Build history of the part. All positions in model axes, mm. Round coordinates to 2 decimals unless told otherwise and drop trailing zeros. Write each loop counter-clockwise with the first axis right and the second up, starting at its lowest first coordinate (ties: lowest second). Pieces come first, ordered by that corner, then holes.
Item 1: Band-saw the part on C-C, the plane x = 142. Write the cut outline in (y, z), then the cut area to 3 significant figures.
Item 2: Drop flat-ended pins along their axis: pin 1 Ø5 at (y, z) = (-13, 14.5) entering from -X; pin 2 Ø3 at (y, z) = (13.5, 13.5) entering from +X. Give the stop position or say it passes through.
Item 3: Wall check: probe 1 along Y at (x, z) = (160, 17); probe 2 along X at (y, z) = (1, 15); probe 3 along X at (y, z) = (-2.5, 13). Give the ranges that are in metal, low to high.
Item 4: Band-saw the part on A-A, the plane x = -160. Write the cut outline in (y, z), then the cut area to 3 significant figures.
Item 5: Band-saw the part on D-D, the plane y = -12.5. Write the cut outline in (x, z), then the cut area to 3 significant figures.
Item 6: Band-saw the part on B-B, the plane z = 15.5. Write the cut outline in (x, y), then the cut area to 3 significant figures.
```python
from build123d import *

# Parameters (mm, degrees)
SKETCH1_W           = 350
SKETCH1_H           = 35
BOSS_EXTRUDE1_DEPTH = 20
SKETCH2_W           = 80
SKETCH2_H           = 20
CUT_EXTRUDE1_DEPTH  = 178.006355818
SKETCH4_R           = 7.5
CUT_EXTRUDE2_DEPTH  = 178.006355818
FILLET1_R           = 10
FILLET2_R           = 10


with BuildPart() as part:
    # Sketch1 → Boss-Extrude1 (new, symmetric)
    with BuildSketch(Plane.XY):
        Rectangle(SKETCH1_W, SKETCH1_H)
    extrude(amount=BOSS_EXTRUDE1_DEPTH, both=True)

    # Sketch2 → Cut-Extrude1 (cut, symmetric)
    with BuildSketch(Plane(origin=(0, 0, 0), x_dir=(1, 0, 0), z_dir=(0, 1, 0))):
        with Locations((-175, 0)):
            Rectangle(SKETCH2_W, SKETCH2_H)
    cut_extrude1 = extrude(amount=CUT_EXTRUDE1_DEPTH, both=True, mode=Mode.SUBTRACT)

    # Sketch4 → Cut-Extrude2 (cut, symmetric)
    with BuildSketch(Plane.XY):
        with Locations((-160, 0)):
            Circle(SKETCH4_R)
    cut_extrude2 = extrude(amount=CUT_EXTRUDE2_DEPTH, both=True, mode=Mode.SUBTRACT)

    # Fillet1
    fillet1_edges = [part.edges().sort_by_distance(p)[0] for p in [
        (-175, -17.5, -15),
        (-175, 17.5, -15),
        (-175, -17.5, 15),
        (-175, 17.5, 15),
    ]]
    fillet(fillet1_edges, radius=FILLET1_R)

    # Mirror3: Cut-Extrude1, Cut-Extrude2 across plane
    add(cut_extrude1.mirror(Plane(origin=(0, 0, 0), x_dir=(0, 0, 1), z_dir=(1, 0, 0))), mode=Mode.SUBTRACT)
    add(cut_extrude2.mirror(Plane(origin=(0, 0, 0), x_dir=(0, 0, 1), z_dir=(1, 0, 0))), mode=Mode.SUBTRACT)

    # Fillet2
    fillet2_edges = [part.edges().sort_by_distance(p)[0] for p in [
        (175, -17.5, -15),
        (175, 17.5, -15),
        (175, -17.5, 15),
        (175, 17.5, 15),
    ]]
    fillet(fillet2_edges, radius=FILLET2_R)


solid = part.part
```
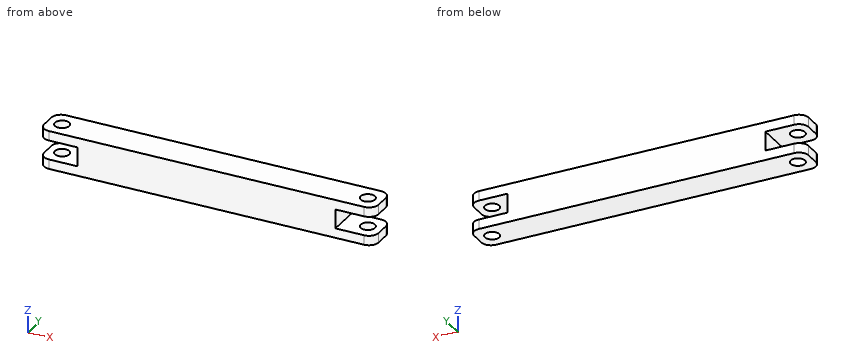
Results:
1. outline: (-17.5, -20) - (17.5, -20) - (17.5, -10) - (-17.5, -10) - close; (-17.5, 10) - (17.5, 10) - (17.5, 20) - (-17.5, 20) - close
1. area: 700 mm2
2. pin 1: stops at x = -174.54
2. pin 2: stops at x = 173.93
3. probe 1: y = -17.5 to -7.5, 7.5 to 17.5
3. probe 2: x = -175 to -167.43, -152.57 to 152.57, 167.43 to 175
3. probe 3: x = -175 to -167.07, -152.93 to 152.93, 167.07 to 175
4. outline: (-17.5, -20) - (-7.5, -20) - (-7.5, -10) - (-17.5, -10) - close; (-17.5, 10) - (-7.5, 10) - (-7.5, 20) - (-17.5, 20) - close; (7.5, -20) - (17.5, -20) - (17.5, -10) - (7.5, -10) - close; (7.5, 10) - (17.5, 10) - (17.5, 20) - (7.5, 20) - close
4. area: 400 mm2
5. outline: (-173.66, -20) - (173.66, -20) - (173.66, -10) - (135, -10) - (135, 10) - (173.66, 10) - (173.66, 20) - (-173.66, 20) - (-173.66, 10) - (-135, 10) - (-135, -10) - (-173.66, -10) - close
5. area: 12,300 mm2
6. outline: (-175, -7.5) arc R10 ccw to (-165, -17.5) - (165, -17.5) arc R10 ccw to (175, -7.5) - (175, 7.5) arc R10 ccw to (165, 17.5) - (-165, 17.5) arc R10 ccw to (-175, 7.5) - close; hole circle Ø15 at (-160, 0); hole circle Ø15 at (160, 0)
6. area: 11,800 mm2
